Geometry: final body of the model. Coordinates: model frame, mm. Give positions to 0.01 mm unless a question says otherwise; leave off trailing zeros. Write each loop counter-clockwise with the first axis right and the second up, starting at its lowest first coordinate (ties: lowest second). Pieces come first, ordered by that corner, then holes.
```python
from build123d import *

# Parameters (mm, degrees)
SKETCH_1_R             = 5.25
SM_BASE_FLANGE_1_DEPTH = 4


# Sheet-metal steps are written as plain solids
with BuildPart() as part:
    # Sketch 1 → Базовая кромка1 (new body)
    with BuildSketch(Plane(origin=(0, 0, 0), x_dir=(1, 0, 0), z_dir=(0, 1, 0))):
        Polygon((-61.091883092, 0), (61.091883092, 0), (61.091883092, 19.091883092), (15, 65.183766184), (-15, 65.183766184), (-61.091883092, 19.091883092), align=None)
        with Locations(Location((-28.5, 32.591883092, 0), (0, 0, 270))):
            Circle(SKETCH_1_R, mode=Mode.SUBTRACT)
        with Locations(Location((-47.591883092, 13.5, 0), (0, 0, 270))):
            Circle(SKETCH_1_R, mode=Mode.SUBTRACT)
        with Locations(Location((47.591883092, 13.5, 0), (0, 0, 90))):
            Circle(SKETCH_1_R, mode=Mode.SUBTRACT)
        with Locations(Location((28.5, 32.591883092, 0), (0, 0, 90))):
            Circle(SKETCH_1_R, mode=Mode.SUBTRACT)
    extrude(amount=-SM_BASE_FLANGE_1_DEPTH)


solid = part.part
```
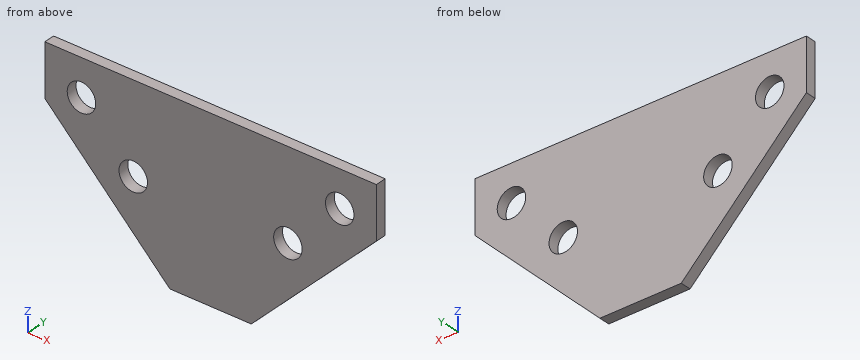
Item 1: Section B-B, the plane x = 28.5. Return the cut outline in (y, z).
Found:
outline: (-4, -51.68) - (0, -51.68) - (0, -37.84) - (-4, -37.84) - close; (-4, -27.34) - (0, -27.34) - (0, 0) - (-4, 0) - close
Item 2: Pin query (flat end, axial travel): pin 1 Ø6.5 at (x, z) = (47.59, -13.5) entering from +Y. Return the tip coordinate at first contact, or that it passes through.
Found:
pin 1: passes through
Item 3: Section C-C, the plane y = -0.6. Return the cut outline in (x, z).
Found:
outline: (-61.09, -19.09) - (-15, -65.18) - (15, -65.18) - (61.09, -19.09) - (61.09, 0) - (-61.09, 0) - close; hole circle Ø10.5 at (-47.59, -13.5); hole circle Ø10.5 at (-28.5, -32.59); hole circle Ø10.5 at (28.5, -32.59); hole circle Ø10.5 at (47.59, -13.5)
Item 4: Section D-D, the plane z = -32. Return the cut outline in (x, y).
Found:
outline: (-48.18, -4) - (-33.72, -4) - (-33.72, 0) - (-48.18, 0) - close; (-23.28, -4) - (23.28, -4) - (23.28, 0) - (-23.28, 0) - close; (33.72, -4) - (48.18, -4) - (48.18, 0) - (33.72, 0) - close
Item 5: Section A-A, the plane z = -13.5. Return the cut outline in (x, y), plus the area to 3 significant figures.
Found:
outline: (-61.09, -4) - (-52.84, -4) - (-52.84, 0) - (-61.09, 0) - close; (-42.34, -4) - (42.34, -4) - (42.34, 0) - (-42.34, 0) - close; (52.84, -4) - (61.09, -4) - (61.09, 0) - (52.84, 0) - close
area: 405 mm2
Item 6: Line query: L1, parallel to X at y = -3.05, z = -13.5; L2, parallel to X at y = -1.05, z = -18; L3, parallel to Z at x = -45.5, y = -1.3. Output: solid intervals per line, ascending.
Found:
L1: x = -61.09 to -52.84, -42.34 to 42.34, 52.84 to 61.09
L2: x = -61.09 to -50.3, -44.89 to 44.89, 50.3 to 61.09
L3: z = -34.68 to -18.32, -8.68 to 0
